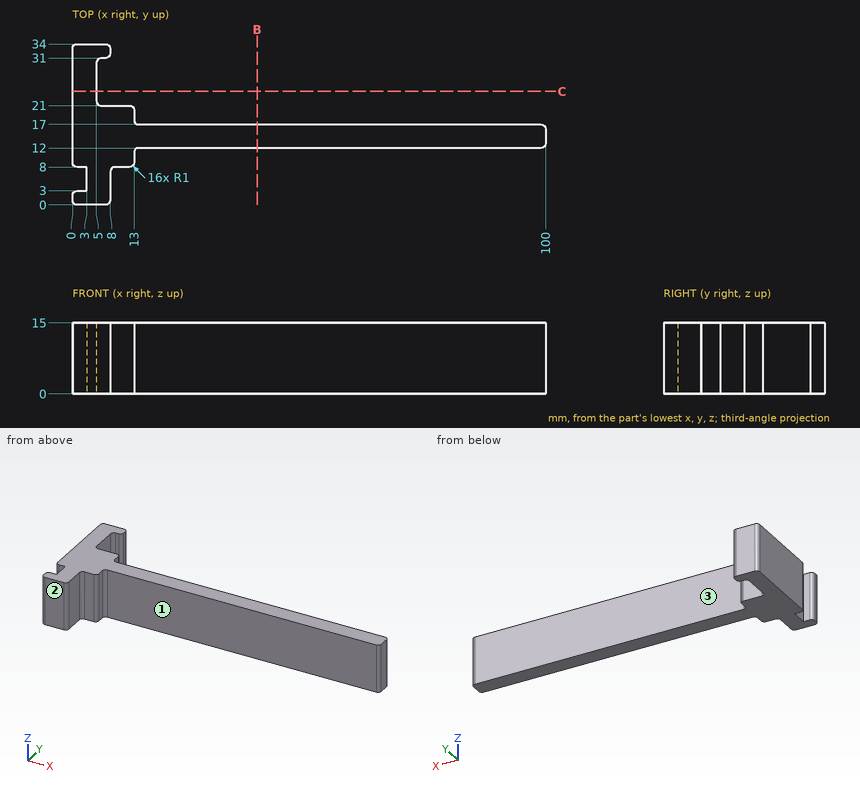
Study the drawing (mm; zero at the part's minimum x, y, z) and answer. A direction names the side the tool comes from. Give positions to 0.01 mm unless a question says otherwise; leave off trailing zeros. Order: outer loops, then holes, each group sorted by start corner. A loop starts at its lowest first (then second) coordinate and runs counter-clockwise, first axis right, second up. Notation, with made-up numbers: (-3, 22) -> (27, 22) arc R22 cw to (27, 30) -> close; hole circle Ø5 at (73.25, -8.5). An arc over 180 degrees is marked (long way). Write item = value, one per line.
1. Straight lines are drawn through the part: line 1 along Y through (x, z) = (20.5, 1.25); line 2 along X through (y, z) = (32.5, 7.5); line 3 along X through (y, z) = (28, 9.25). For each, find the intervals that lie inside material, in ascending order.
Numbers:
line_1 = 12 to 17
line_2 = 0 to 8
line_3 = 0 to 5
2. For the marked faces 1, 2 and 3, determine the directions among +Z, -Z, +X, -X, +Y, -Y from which every point of the face is accessible in a straight line to the end or side of a thin tool.
Numbers:
face_1 = +Z, -Z, +X, -Y
face_2 = +Z, -Z, +X, -X, -Y
face_3 = +Z, -Z, +X, +Y
3. A cutting plane is placed at B-B, the plane x = 39. Write down the section's boundary in (y, z).
Numbers:
outline = (12, 0) -> (17, 0) -> (17, 15) -> (12, 15) -> close
4. A cutting plane is placed at C-C, the plane y = 24. Write down the section's boundary in (x, z).
Numbers:
outline = (0, 0) -> (5, 0) -> (5, 15) -> (0, 15) -> close
5. Given pin 1 (5 mm diameter, centred on y = 5, z = 4, fed in from +X); pin 2 (7.5 mm diameter, centred on x = 58, z = 6, fed in from +Y); pin 3 (4 mm diameter, centred on y = 6.5, z = 6, fed in from -X), each flat-ended and moving along its own axis, determine where each tip first touches the part or whether it passes through.
Numbers:
pin_1 = 8.13
pin_2 = 17
pin_3 = 0.13
